The listing builds one solid part. Answer for the finished solid, in the listing's coordinates (mm). A direction names the side the tool comes from. Round coordinates to 2 decimals unless told otherwise and drop trailing zeros. Loops run counter-clockwise (first coordinate to the right, second up) from the corner with the lowest first, then second, coordinate; pieces in that order, holes last. Notation, with made-up numbers: (-28.75, 67) -> (-1.75, 67) arc R27 cw to (-1.75, 83) -> close; hole circle Ø2 at (17.5, -14.75). An arc over 180 degrees is marked (long way). Answer in a Markdown table with one row per item. Add a question column.
```python
from build123d import *

# Parameters (mm, degrees)
PAD_DEPTH   = 40
SKETCH001_R = 3.3
HOLE_DEPTH  = 3.001


with BuildPart() as part:
    # Sketch → Pad (new body, symmetric)
    with BuildSketch(Plane.YZ):
        with BuildLine():
            Line((0, 25), (0, 0))
            Line((0, 0), (-25, 0))
            Line((-25, 0), (-25, 1.25))
            ThreePointArc((-23.25, 3), (-24.487437, 2.487437), (-25, 1.25))
            Line((-23.25, 3), (-6.5, 3))
            ThreePointArc((-6.5, 3), (-4.025126, 4.025126), (-3, 6.5))
            Line((-3, 6.5), (-3, 23.25))
            ThreePointArc((-1.25, 25), (-2.487437, 24.487437), (-3, 23.25))
            Line((0, 25), (-1.25, 25))
        make_face()
    extrude(amount=PAD_DEPTH, both=True)

    # Sketch001 (on Face6 of Pad) → Hole (cut, through all)
    with BuildSketch(Plane(origin=(0, 0, 3), x_dir=(0, -1, 0), z_dir=(0, 0, 1))):
        with Locations((15, 30)):
            Circle(SKETCH001_R)
        with Locations((15, -30)):
            Circle(SKETCH001_R)
    extrude(amount=-HOLE_DEPTH, mode=Mode.SUBTRACT)


solid = part.part
```
Item 1: Section A-A, the plane x = -30 is taken. Write down the section's boundary in (y, z), and give its area (3 significant figures).
Item 2: Consider L1, parallel to X at y = -15, z = 1.6; L2, parallel to X at y = -15.75, z = 2.75; L3, parallel to Y at x = 16.5, z = 16.5. Determine where each line is inside the solid, lowest interval first. Write a range as from..to.
Item 3: Section B-B, the plane y = -15 is taken. Write down the section's boundary in (x, z), and give its area (3 significant figures).
Item 4: The mould has two halves that part along X. Classify faces 1 (the cylindrical face through (32.23, -12.57, 1.52)), 2 (the flat face through (-40, -3, 5)), 3 (the flat face through (40, -3, 5)): +X half, -X half, draft (parallel to the pull), parting line (faces both ways), or undercut.
Item 5: For faces 4 (the flat face through (1, -3, 15)), 5 (the flat face through (1, 0, 13)), determine the directions among +Z, -Z, +X, -X, +Y, -Y from which every point of the face is accessible in a straight line to the end or side of a thin tool.
Item 6: Section C-C, the plane x = 35.5 is taken. Write down the section's boundary in (y, z), and give its area (3 significant figures).
Item 7: Flat-ended cylindrical pins translate along their axes: P1, Ø13.5, axis at x = 19, z = 12.5, coming from the -Y side; P2, Ø8, axis at x = -9.5, z = 17, coming from the -Y side; P3, Ø6, axis at x = 30, y = -15, coming from the -Z side; P4, Ø13.5, axis at x = -19, y = -14, coming from the +Z side. Find the tip coordinate at first contact, or state that the pin passes through.
Item 8: Section D-D, the plane z = 15 is taken. Write down the section's boundary in (x, y).
Here are the results:
| question | item | result |
|---|---|---|
| 1 | outline | (-25, 0) -> (-18.3, 0) -> (-18.3, 3) -> (-23.25, 3) arc R1.75 ccw to (-25, 1.25) -> close; (-11.7, 0) -> (0, 0) -> (0, 25) -> (-1.25, 25) arc R1.75 ccw to (-3, 23.25) -> (-3, 6.5) arc R3.5 cw to (-6.5, 3) -> (-11.7, 3) -> close |
| 1 | area | 123 mm² |
| 2 | L1 | x = -40..-33.3, -26.7..26.7, 33.3..40 |
| 2 | L2 | x = -40..-33.21, -26.79..26.79, 33.21..40 |
| 2 | L3 | y = -3..0 |
| 3 | outline | (-40, 0) -> (-33.3, 0) -> (-33.3, 3) -> (-40, 3) -> close; (-26.7, 0) -> (26.7, 0) -> (26.7, 3) -> (-26.7, 3) -> close; (33.3, 0) -> (40, 0) -> (40, 3) -> (33.3, 3) -> close |
| 3 | area | 200 mm² |
| 4 | face 1 | undercut |
| 4 | face 2 | -X half |
| 4 | face 3 | +X half |
| 5 | face 4 | +Z, +X, -X, -Y |
| 5 | face 5 | +Z, -Z, +X, -X, +Y |
| 6 | outline | (-25, 0) -> (0, 0) -> (0, 25) -> (-1.25, 25) arc R1.75 ccw to (-3, 23.25) -> (-3, 6.5) arc R3.5 cw to (-6.5, 3) -> (-23.25, 3) arc R1.75 ccw to (-25, 1.25) -> close |
| 6 | area | 142 mm² |
| 7 | P1 | stops at y = -3.08 |
| 7 | P2 | stops at y = -3 |
| 7 | P3 | passes through |
| 7 | P4 | stops at z = 3 |
| 8 | outline | (-40, -3) -> (40, -3) -> (40, 0) -> (-40, 0) -> close |
